Autodesk Inventor part; units mm, degrees
ref_plane "YZ Plane" through (0, 0, 0) normal (1, 0, 0) x (0, 1, 0)
ref_plane "XZ Plane" through (0, 0, 0) normal (0, 1, 0) x (-1, 0, 0)
ref_plane "XY Plane" through (0, 0, 0) normal (0, 0, 1) x (1, 0, 0)
sketch "Sketch1" plane through (0, 0, 0) normal (0, 0, 1) x (1, 0, 0)
  line L0 (0, 0) -> (150, 0)
  line L1 (150, 0) -> (150, 100)
  line L2 (150, 100) -> (0, 100)
  line L3 (0, 100) -> (0, 0)
  line L4 (5, 5) -> (145, 5)
  line L5 (145, 5) -> (145, 95)
  line L6 (145, 95) -> (5, 95)
  line L7 (5, 95) -> (5, 5)
  circle A0 centre (37.5, 60) radius 5
  line L8 (5, 60) -> (145, 60) construction
  circle A1 centre (72.5, 60) radius 5
  circle A2 centre (107.5, 60) radius 5
  arc A3 (10, 17) -> (17, 10) centre (17, 17) ccw
  arc A4 (57, 10) -> (60.71, 22.936) centre (57, 17) ccw
  arc A5 (20.71, 47.936) -> (10, 42) centre (17, 42) ccw
  line L9 (17, 10) -> (57, 10)
  line L10 (20.71, 47.936) -> (60.71, 22.936)
  line L11 (10, 17) -> (10, 42)
  circle A6 centre (130, 25) radius 8
  circle A7 centre (90, 25) radius 8
  line L12 (90, 25) -> (145, 25) construction
  arc A8 (124.2857, 19.4012) -> (95.7143, 19.4012) centre (110, 5.4041) ccw
  arc A9 (90.0041, 5) -> (90.0154, 4.6201) centre (110, 5.4041) ccw
  arc A10 (135.7143, 30.5988) -> (84.2857, 30.5988) centre (110, 5.4041) ccw
  dimension "d0" = 150
  dimension "d1" = 100
  dimension "d2" = 140
  dimension "d19" = 35
  dimension "d25" = 17
  dimension "d26" = 17
  dimension "d28" = 40
  dimension "d30" = 25
  dimension "d31" = 16
  dimension "d32" = 25
  dimension "d33" = 20
  dimension "d34" = 40
  dimension "d35" = 25
  dimension "d102" = 5
  dimension "d103" = 5
  dimension "d104" = 40
  dimension "d106" = 37.5
  dimension "d107" = 10
  dimension "d108" = 20
  dimension "d109" = 5
  dimension "d111" = 36
  dimension "d112" = 7
  dimension "d113" = 7
  dimension "d115" = 16
  dimension "d116" = 10
  dimension "d120" = 47.1699
  dimension "d121" = 40
extrude "Extrusion1" add sketch "Sketch1" against normal blind 40 contours L3 L2 L1 L0 | L7 L6 L5 L4 | A0 | A1 | A2 | L11 A5 L10 A4 L9 A3 | A6 | A6 A8 A7 A10 | A7
extrude "Extrusion2" add sketch "Sketch1" along normal blind 10 contours L7 L6 L5 L4
extrude "Extrusion3" add sketch "Sketch1" along normal blind 10 contours A0 | A1 | A2
hole "Hole1" at (37.5, 60, 0) direction (0, 0, 1) diameter 10 end through all
hole "Hole2" at (72.5, 60, 0) direction (0, 0, 1) diameter 10 end through all
hole "Hole3" at (107.5, 60, 0) direction (0, 0, 1) diameter 10 end through all
hole "Hole4" at (37.5, 60, 0) direction (0, 0, -1) diameter 10 depth 13 tip angle 118
hole "Hole5" at (72.5, 60, 0) direction (0, 0, -1) diameter 10 depth 13 tip angle 118
hole "Hole6" at (107.5, 60, 0) direction (0, 0, -1) diameter 10 depth 13 tip angle 118
fillet "Fillet1" radius 5 1 edges at (145, 95, 5)
fillet "Fillet2" radius 5 3 edges at (5, 95, 5) (145, 5, 5) (5, 5, 5)
sketch "Sketch2" plane through (0, 0, 10) normal (0, 0, 1) x (1, 0, 0)
  arc A0 (30, 80) -> (10, 80) centre (20, 80) ccw
  line L0 (0, 100) -> (0, 0)
  line L1 (5, 10) -> (5, 90) construction
  line L2 (5, 80) -> (145, 80) construction
  line L3 (145, 90) -> (145, 10) construction
  line L4 (10, 80) -> (30, 80)
  arc A1 (65, 80) -> (45, 80) centre (55, 80) ccw
  line L5 (45, 80) -> (65, 80)
  arc A2 (100, 80) -> (80, 80) centre (90, 80) ccw
  line L6 (80, 80) -> (100, 80)
  arc A3 (135, 80) -> (115, 80) centre (125, 80) ccw
  line L7 (115, 80) -> (135, 80)
  dimension "d90" = 20
  dimension "d122" = 80
  dimension "d131" = 20
  dimension "d132" = 10
  dimension "d135" = 35
revolve "Revolution1" add sketch "Sketch2" angle 360 about axis through (5, 80, 10) along (1, 0, 0)
chamfer "Chamfer1" distance 2 angle 45 4 edges at (75, 100, 0) (150, 50, 0) (0, 50, 0) (75, 0, 0)
properties part number "tarefa 3"
Verification items for the finished model (mm, model axes). A direction names the side the tool comes from. Coordinates: 2 decimals unless noted, no trailing zeros. Loops run counter-clockwise (first coordinate to the right, second up) from the corner with the lowest first, then second, coordinate; pieces in that order, holes last. Notation, with made-up numbers: M 44,25 L 86,25 A23 cw 86,34 Z; hole C -15.75,-36 d2. An arc over 180 degrees is marked long. One line per item, written item: value.
1. Section check C-C on y = 14.5. Record the cut outline in (x, z).
Answers follow:
outline: M 0,-40 L 150,-40 L 150,-2 L 148,0 L 145,0 L 145,10 L 63.54,10 L 63.54,0 L 10.46,0 L 10.46,10 L 5,10 L 5,0 L 2,0 L 0,-2 Z
2. Mould release check, pull along X, two halves, no side actions. Record for faces 1 (the cylindrical face through (6, 7, 5)), 2 (the cylindrical face through (144, 93, 5)), 3 (the cylindrical face through (13.516, 48.071, 4.93)): pulls with the +X half, pulls with the -X half, needs draft (parallel to the pull), parting line crosses it, or undercut.
Answers follow:
face 1: pulls with the -X half
face 2: pulls with the +X half
face 3: undercut
3. Set-up check for faces 4 (the cylindrical face through (143, 6, 5)), 5 (the cylindrical face through (7, 94, 5)), 6 (the flat face through (110, 29, 0)): record each of +Z, -Z, +X, -X, +Y, -Y from which the full face is reachable in a straight line by a thin tool's end or side.
Answers follow:
face 4: +Z, +X, -Y
face 5: +Z, -X, +Y
face 6: +Z
4. Section check B-B on x = 12. Record the cut outline in (y, z), plus the area to 3 significant figures.
Answers follow:
outline: M 0,-40 L 100,-40 L 100,-2 L 98,0 L 95,0 L 95,10 L 86,10 A6 ccw 74,10 L 46.9,10 L 46.9,0 L 12.1,0 L 12.1,10 L 5,10 L 5,0 L 2,0 L 0,-2 Z
area: 4,600 mm^2
5. Material ranges on line 1 along X through (y, z) = (60, 4); line 2 along X through (y, z) = (60, -2.25); line 3 along Y through (x, z) = (107, -7), recorded low to high. Write a range as from..to.
Answers follow:
line 1: 5..32.5, 42.5..67.5, 77.5..102.5, 112.5..145
line 2: 0..32.5, 42.5..67.5, 77.5..102.5, 112.5..150
line 3: 0..55.03, 64.97..100
6. Gauge pin test, flat ends, axial feed: P1, Ø5, axis at x = 98, z = 3, coming from the +Y side; P2, Ø11.5, axis at x = 107.5, y = 60, coming from the +Z side; P3, Ø3, axis at y = 39, z = 6.5, coming from the -X side. Record the tip position at first contact, or that the pin passes through.
Answers follow:
P1: y = 95
P2: z = 10
P3: x = 5
7. Section check D-D on x = 130. Record the cut outline in (y, z).
Answers follow:
outline: M 0,-40 L 100,-40 L 100,-2 L 98,0 L 95,0 L 95,10 L 88.66,10 A8.66 ccw 71.34,10 L 35.34,10 L 35.34,0 L 17,0 L 17,10 L 5,10 L 5,0 L 2,0 L 0,-2 Z
8. Section check A-A on z = 8. Record the cut outline in (x, y), plus the area to 3 significant figures.
Answers follow:
outline: M 5,10 A5 ccw 10,5 L 140,5 A5 ccw 145,10 L 145,90 A5 ccw 140,95 L 10,95 A5 ccw 5,90 Z; hole M 10,17 A7 ccw 17,10 L 57,10 A7 ccw 60.71,22.94 L 20.71,47.94 A7 ccw 10,42 Z; hole C 37.5,60 d10; hole C 72.5,60 d10; hole M 84.29,30.6 A8 ccw 95.71,19.4 A20 cw 124.29,19.4 A8 ccw 135.71,30.6 A36 ccw Z; hole C 107.5,60 d10
area: 9,990 mm^2
